Build history of the part. All positions in model axes, mm. A direction names the side the tool comes from. Give positions to 0.01 mm unless a question says otherwise; leave off trailing zeros. Write each loop counter-clockwise with the first axis right and the second up, starting at its lowest first coordinate (ties: lowest second). Pieces come first, ordered by that corner, then holes. Notation, with made-up numbers: (-11.75, -38.75) - (27.25, -38.75) arc R8 cw to (27.25, -30.75) - close; hole circle Ø8 at (9, 0.5). An arc over 180 degrees is marked (long way). Use one line per item in the form item = value. Start each with the question number.
Autodesk Inventor part; units mm, degrees
ref_plane "YZ Plane" through (0, 0, 0) normal (1, 0, 0) x (0, 1, 0)
ref_plane "XZ Plane" through (0, 0, 0) normal (0, 1, 0) x (-1, 0, 0)
ref_plane "XY Plane" through (0, 0, 0) normal (0, 0, 1) x (1, 0, 0)
sketch "Sketch1" plane through (0, 0, 0) normal (0, 1, 0) x (-1, 0, 0)
  line L0 (-13, 0) -> (0, 0)
  line L1 (0, 0) -> (0, 3)
  line L2 (0, 3) -> (-13, 3)
  line L3 (-13, 3) -> (-13, 0)
  line L4 (-13, 3) -> (-10, 3)
  line L5 (-10, 3) -> (-10, 19)
  line L6 (-10, 19) -> (-13, 19)
  line L7 (-13, 19) -> (-13, 3)
  line L8 (0, 3) -> (-3, 3)
  line L9 (-3, 3) -> (-3, 19)
  line L10 (-3, 19) -> (0, 19)
  line L11 (0, 19) -> (0, 3)
  point P0 (0, 0)
  dimension "d0" = 13
  dimension "d1" = 3
  dimension "d2" = 3
  dimension "d3" = 16
  dimension "d4" = 3
  dimension "d5" = 16
extrude "Extrusion1" add sketch "Sketch1" along normal blind 3
(1) Cut at C-C, the plane x = 9. Give the cut face in (y, z), then the cut area to 3 significant figures.
(2) Pin check, flat tip, straight feed: pin 1 Ø1.5 at (x, y) = (6.5, 1.5) entering from +Z. Stop position of the tip, or through.
(3) Wall check: line 1 (X direction, y = 2.55, z = 10.5); line 2 (Z direction, x = 6.5, y = 1.8). Give the ranges that are in metal, low to high. Write a range as from..to.
(4) Cut at A-A, the plane z = 17.25. Give the cut face in (x, y).
(5) Which spindle directions (+Z, -Z, +X, -X, +Y, -Y) get a long thin tool onto all of the face, cutting with end or side? Do faces 1 (the flat face through (2, 0, 10)), 2 (the flat face through (3, 1, 11)). Say none if no direction does.
(6) Cut at B-B, the plane y = 1.3. Give the cut face in (x, z), then the cut area to 3 significant figures.
(7) Two-plate mould, pull along X, no slides. Class faces 3 (the flat face through (13, 1, 10)), 4 (the flat face through (2, 1, 19)), 5 (the flat face through (6, 1, 3)), 6 (the flat face through (0, 1, 9)): +X half, -X half, draft (parallel to the pull), parting line (faces both ways), or undercut.
Solution:
q1.outline = (0, 0) - (3, 0) - (3, 3) - (0, 3) - close
q1.area = 9.00 mm2
q2.pin_1 = 3
q3.line_1 = 0..3, 10..13
q3.line_2 = 0..3
q4.outline = (0, 0) - (3, 0) - (3, 3) - (0, 3) - close; (10, 0) - (13, 0) - (13, 3) - (10, 3) - close
q5.face_1 = +Z, -Z, +X, -X, -Y
q5.face_2 = +Z, +Y, -Y
q6.outline = (0, 0) - (13, 0) - (13, 19) - (10, 19) - (10, 3) - (3, 3) - (3, 19) - (0, 19) - close
q6.area = 135 mm2
q7.face_3 = +X half
q7.face_4 = draft
q7.face_5 = undercut
q7.face_6 = -X half
